Check sheet for the drawn part. Datum: minimum x, y, z corner. Units: mm. Give positions to 0.01 mm unless a question says otherwise; leave off trailing zeros. Order: outer loops, then holes, each group sorted by start corner. A loop starts at its lowest first (then second) coordinate and runs counter-clockwise, first axis right, second up. Notation, with made-up numbers: M 17.5,78.25 L 47.5,78.25 A35 cw 47.5,113.25 Z; hole C -4.5,44 d2. An arc over 180 degrees is marked long. Answer as CSV lines item,"result". Start each with the question number.
Q1. Section check A-A, the plane x = 48. Record the boundary of the cut face in (y, z).
Q2. Thickness scan on line 1 (X direction, y = 0.2, z = 23.5); line 2 (X direction, y = 0.3, z = 49.5); line 3 (Z direction, x = 46.2, y = 0.9). Record the ranges inside material, lowest first.
Q3. Section check B-B, the plane z = 45. Record the boundary of the cut face in (x, y), then the cut area to 3 significant figures.
Q4. Section check C-C, the plane y = 1.1. Count the separate pieces of the cut face and the enclosed holes in it, then the cut area to 3 significant figures.
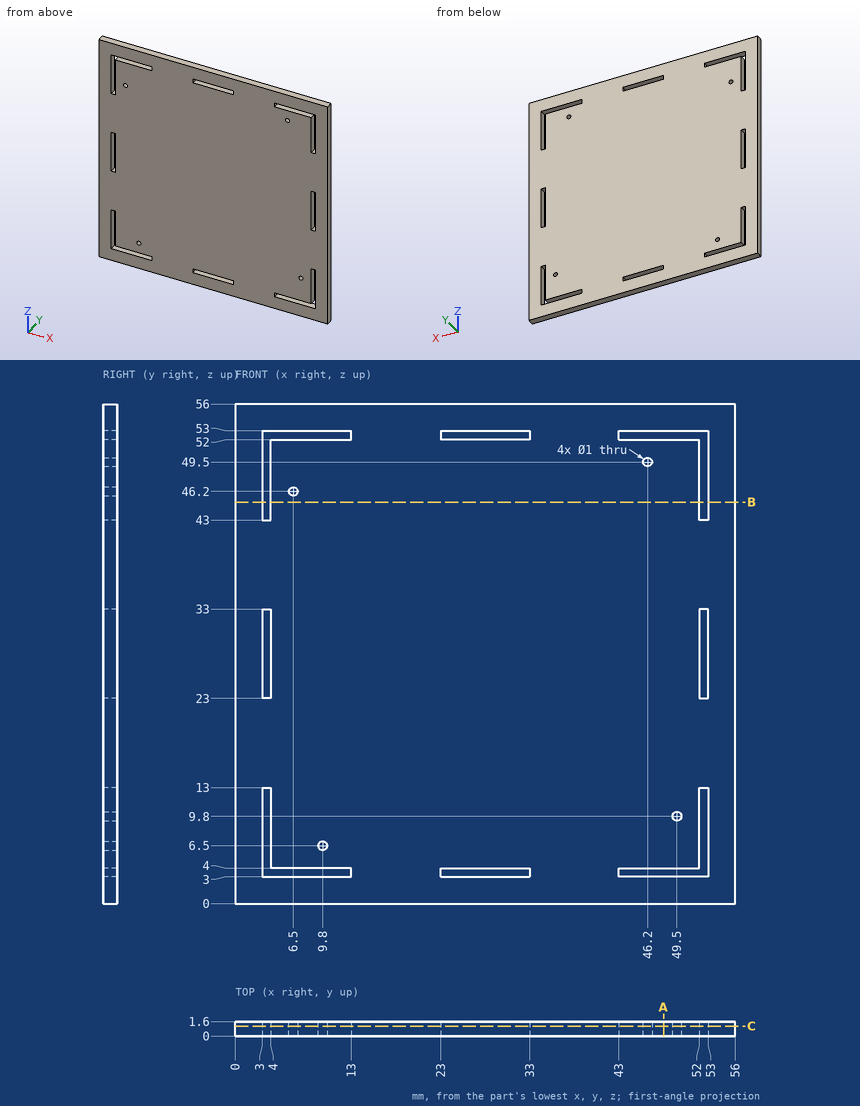
Answer block:
1,outline,"M 0,0 L 1.6,0 L 1.6,3 L 0,3 Z; M 0,4 L 1.6,4 L 1.6,52 L 0,52 Z; M 0,53 L 1.6,53 L 1.6,56 L 0,56 Z"
2,line 1,"x = 0 to 3, 4 to 52, 53 to 56"
2,line 2,"x = 0 to 3, 4 to 45.7, 46.7 to 52, 53 to 56"
2,line 3,"z = 0 to 3, 4 to 49, 50 to 52, 53 to 56"
3,outline,"M 0,0 L 3,0 L 3,1.6 L 0,1.6 Z; M 4,0 L 52,0 L 52,1.6 L 4,1.6 Z; M 53,0 L 56,0 L 56,1.6 L 53,1.6 Z"
3,area,"86.4 mm2"
4,separate pieces,"1"
4,enclosed holes,"12"
4,area,"3,020 mm2"
